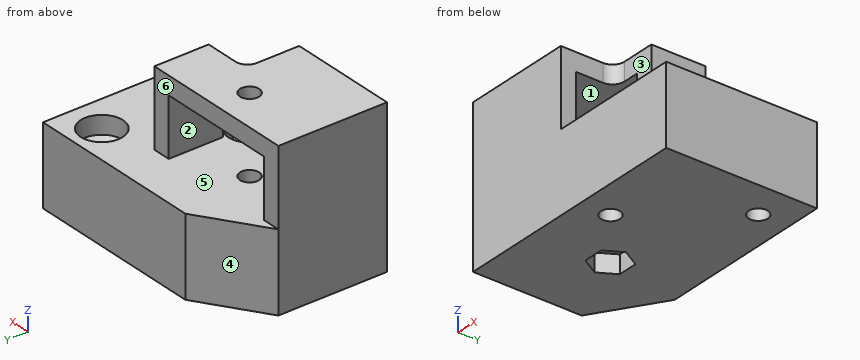
```python
from build123d import *

# Parameters (mm, degrees)
SKETCH_1_W                  = 12.6
SKETCH_1_H                  = 9
EXTRUDE_1_DEPTH             = 3
SKETCH_2_W                  = 3
SKETCH_2_H                  = 9
EXTRUDE_2_DEPTH             = 20
SKETCH_3_W                  = 12.6
SKETCH_3_H                  = 9
EXTRUDE_3_DEPTH             = 3
EXTRUDE_4_DEPTH             = 6.5
SKETCH_5_W                  = 18.4
SKETCH_5_H                  = 12.6
EXTRUDE_5_DEPTH             = 2.5
SKETCH_6_W                  = 40.5
SKETCH_6_H                  = 25
EXTRUDE_6_DEPTH             = 13
CUT_EXTRUDE_1_DEPTH         = 3
HOLE_WIZARD_M31_AT_2_COUNT  = 2
HOLE_WIZARD_M31_AT_2_PITCH  = 19.209372712
SKETCH_10_W                 = 1.6
SKETCH_10_H                 = 13
HOLE_WIZARD_3_2_3_2_2_D     = 3.2
HOLE_WIZARD_3_2_3_2_2_DEPTH = 25.6
CHAMFER_1_SIZE              = 6.981980506
CHAMFER_1_SIZE2             = 10.66515139
FILLET_1_R                  = 2


with BuildPart() as part:
    # Эскиз1 → Бобышка-Вытянуть1 (new body)
    with BuildSketch(Plane(origin=(272.1, 0, 0), x_dir=(0, 0, -1), z_dir=(1, 0, 0))):
        with Locations((-16.8, 19.5)):
            Rectangle(SKETCH_1_W, SKETCH_1_H)
    extrude(amount=-EXTRUDE_1_DEPTH)

    # Эскиз2 → Бобышка-Вытянуть2 (add)
    with BuildSketch(Plane.ZY.offset(-269.1)):
        with Locations((21.6, 19.5)):
            Rectangle(SKETCH_2_W, SKETCH_2_H)
    extrude(amount=EXTRUDE_2_DEPTH)

    # Эскиз3 → Бобышка-Вытянуть3 (add)
    with BuildSketch(Plane.ZY.offset(-249.1)):
        with Locations((16.8, 19.5)):
            Rectangle(SKETCH_3_W, SKETCH_3_H)
    extrude(amount=EXTRUDE_3_DEPTH)

    # Эскиз4 → Бобышка-Вытянуть4 (add)
    with BuildSketch(Plane.XZ.offset(-15)):
        Polygon((264.5, 23.1), (264.5, 20.1), (249.1, 20.1), (249.1, 10.5), (246.1, 10.5), (246.1, 23.1), align=None)
    extrude(amount=EXTRUDE_4_DEPTH)

    # Эскиз5 → Бобышка-Вытянуть5 (add)
    with BuildSketch(Plane.XZ.offset(-8.5)):
        with Locations((255.3, 16.8)):
            Rectangle(SKETCH_5_W, SKETCH_5_H)
    extrude(amount=EXTRUDE_5_DEPTH)

    # Эскиз6 → Бобышка-Вытянуть6 (add)
    with BuildSketch(Plane(origin=(0, 0, 10.5), x_dir=(-1, 0, 0), z_dir=(0, 0, -1))):
        with Locations((-266.35, 18.5)):
            Rectangle(SKETCH_6_W, SKETCH_6_H)
    extrude(amount=EXTRUDE_6_DEPTH)

    # Эскиз7 → Вырез-Вытянуть1 (cut)
    with BuildSketch(Plane(origin=(0, 0, -2.5), x_dir=(-1, 0, 0), z_dir=(0, 0, -1))):
        Polygon((-257.454551733, 15.65), (-255.809103466, 18.5), (-257.454551733, 21.35), (-260.745448267, 21.35), (-262.390896534, 18.5), (-260.745448267, 15.65), align=None)
    extrude(amount=-CUT_EXTRUDE_1_DEPTH, mode=Mode.SUBTRACT)

    # Эскиз8 → Зенковка для  винта с плоской головкой M31 (revolve, cut)
    with BuildSketch(Plane(origin=(280.6, 26, 10.5), x_dir=(0, -1, 0), z_dir=(1, 0, 0))):
        Polygon((0, 0), (0, 13), (1.6, 13), (1.6, 4.141635176), (3.5, 3), (3.5, 0), align=None)
    hole_wizard_m31 = revolve(axis=Axis((280.6, 26, 16.85), (0, 0, -1)), mode=Mode.SUBTRACT)

    # Зенковка для  винта с плоской головкой M31 at 2: Зенковка для  винта с плоской головкой M31 ×2
    with Locations(*[Vector(-0.6246950475544251, -0.7808688094430297, 0) * (i * HOLE_WIZARD_M31_AT_2_PITCH) for i in range(1, HOLE_WIZARD_M31_AT_2_COUNT)]):
        add(hole_wizard_m31, mode=Mode.SUBTRACT)

    # Эскиз10 → Диаметр отверстия Ø3.2 (3.2)1 (revolve, cut)
    with BuildSketch(Plane(origin=(259.1, 18.5, 10.5), x_dir=(0, -1, 0), z_dir=(1, 0, 0))):
        with Locations((0.8, 6.5)):
            Rectangle(SKETCH_10_W, SKETCH_10_H)
    revolve(axis=Axis((259.1, 18.5, 16.85), (0, 0, -1)), mode=Mode.SUBTRACT)

    # Диаметр отверстия Ø3.2 (3.2)2
    with Locations(Plane.XY.offset(23.1)):
        with Locations((259.1, 18.5)):
            Hole(HOLE_WIZARD_3_2_3_2_2_D / 2, depth=HOLE_WIZARD_3_2_3_2_2_DEPTH)

    # Фаска1
    chamfer_1_edges = [part.edges().sort_by_distance(p)[0] for p in [
        (246.1, 31, 4),
    ]]
    chamfer_1_side = [part.faces().sort_by_distance(p)[0] for p in [
        (246.1, 17.061435303, 9.261036607),
    ]]
    chamfer(chamfer_1_edges, length=CHAMFER_1_SIZE, length2=CHAMFER_1_SIZE2, reference=chamfer_1_side[0])

    # Скругление1
    fillet_1_edges = [part.edges().sort_by_distance(p)[0] for p in [
        (264.5, 15, 21.6),
        (249.1, 8.5, 15.3),
    ]]
    fillet(fillet_1_edges, radius=FILLET_1_R)


solid = part.part
```
Can you work these out from the model? Positions are in its coordinate system, mm. Face numbers are marked on the shaded views. A direction names the side the tool comes from. Coordinates: 2 decimals unless noted, no trailing zeros. Loops run counter-clockwise (first coordinate to the right, second up) from the corner with the lowest first, then second, coordinate; pieces in that order, holes last. Notation, with made-up numbers: M 73,-25.5 L 122,-25.5 A11 cw 122,-16.5 Z; hole C 75.25,86 d9. An arc over 180 degrees is marked long. Put each result on its own line as item: value. Start each with the question number.
(1) I need wall thicknesses on probe 1 along Z at (x, y) = (261, 18.5); probe 2 along X at (y, z) = (23.5, 12); probe 3 along Z at (x, y) = (263, 16). Which ranges of each line are inside material? Lowest first, please.
(2) We'd pull the mould along X, two halves only. Please class the marked faces 4, 5 and 6: +X half, -X half, draft (parallel to the pull), parting line (faces both ways), or undercut.
(3) Imagine slicing it at D-D on x = 280.6. List the corners of the cut face in (y, z) for me.
(4) Imagine slicing it at B-B on z = 21. List the corners of the cut face in (x, y) for me.
(5) Which directions (+Z, -Z, +X, -X, +Y, -Y) give clear straight access to the entire face, cutting with the end or side of a thin tool? Please do the marked faces 1, 2 and 3.
(6) Imagine slicing it at C-C on y = 11. List the corners of the cut face in (x, z) for me, and give its area (3 significant figures).
(7) Imagine slicing it at A-A on x = 268.6. List the corners of the cut face in (y, z) for me, and give its area (3 significant figures).
(8) Will these pins go through, and if not, where does the flat tip stop? pin 1 Ø2.5 at (x, y) = (259.1, 18.5) entering from +Z; pin 2 Ø6 at (x, z) = (265.5, 14.5) entering from +Y; pin 3 Ø1.7 at (x, y) = (258.5, 20) entering from -Z; pin 4 Ø11 at (x, y) = (280.6, 26) entering from -Z.
Worked answers:
1. probe 1: z = 0.5 to 10.5, 20.1 to 23.1
1. probe 2: x = 246.1 to 249.1, 269.1 to 272.1
1. probe 3: z = -2.5 to 10.5, 20.1 to 23.1
2. face 4: -X half
2. face 5: undercut
2. face 6: draft
3. outline: M 6,-2.5 L 24.4,-2.5 L 24.4,6.36 L 22.5,7.5 L 22.5,10.5 L 6,10.5 Z; M 27.6,-2.5 L 31,-2.5 L 31,10.5 L 29.5,10.5 L 29.5,7.5 L 27.6,6.36 Z
4. outline: M 246.1,6 L 264.5,6 L 264.5,13 A2 cw 266.5,15 L 272.1,15 L 272.1,24 L 246.1,24 Z; hole C 259.1,18.5 d3.2
5. face 1: +Y
5. face 2: +Y, -Y
5. face 3: +Z, +X, -Y
6. outline: M 246.1,-2.5 L 267,-2.5 L 267,6.36 L 265.1,7.5 L 265.1,10.5 L 249.1,10.5 L 249.1,20.1 L 264.5,20.1 L 264.5,23.1 L 246.1,23.1 Z; M 270.2,-2.5 L 286.6,-2.5 L 286.6,10.5 L 272.1,10.5 L 272.1,7.5 L 270.2,6.36 Z
6. area: 555 mm2
7. outline: M 6,-2.5 L 9.4,-2.5 L 9.4,6.36 L 7.5,7.5 L 7.5,10.5 L 6,10.5 Z; M 12.6,-2.5 L 31,-2.5 L 31,10.5 L 14.5,10.5 L 14.5,7.5 L 12.6,6.36 Z; M 15,20.1 L 24,20.1 L 24,23.1 L 15,23.1 Z
7. area: 297 mm2
8. pin 1: passes through
8. pin 2: stops at y = 8.5
8. pin 3: stops at z = 0.5
8. pin 4: stops at z = -2.5
